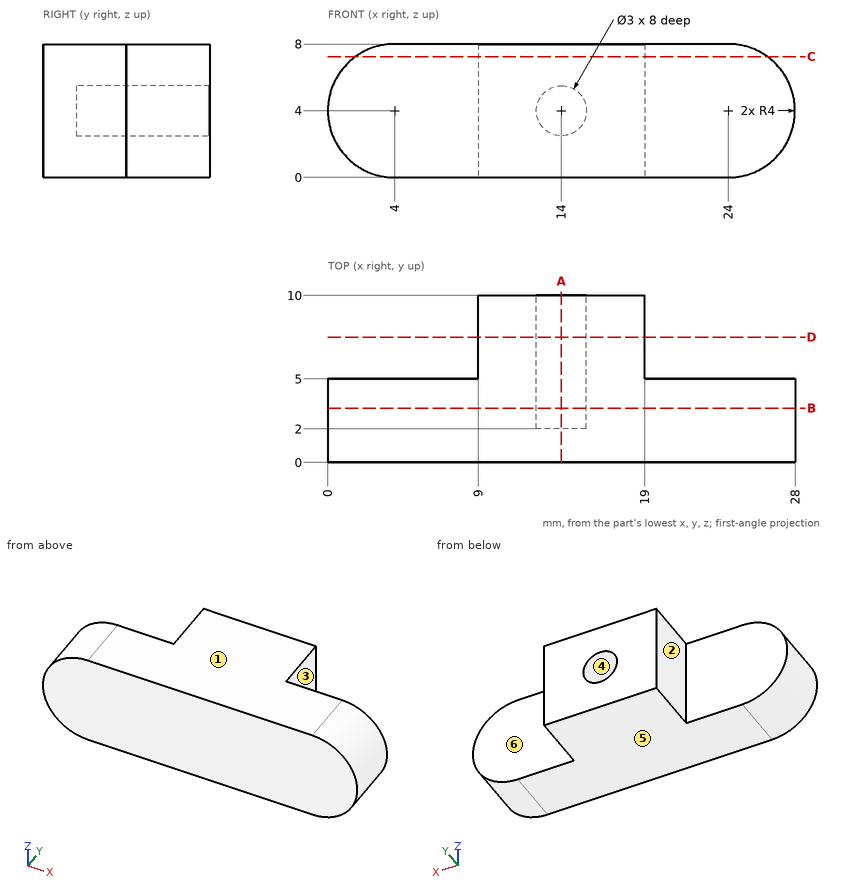
Input: dimensioned drawing with shaded views. Units: mm. Origin: part minimum x, y, z. A direction names the side the tool comes from. Coordinates: 2 decimals unless noted, no trailing zeros. Order: outer loops, then holes, each group sorted by start corner. A loop starts at its lowest first (then second) coordinate and runs counter-clockwise, first axis right, second up. Notation, with made-up numbers: M 58.5,18 L 63.5,18 A26 cw 63.5,48 Z; hole C 4.5,-16 d8. An arc over 180 degrees is marked long. Write each question's results on one line, items separated by ' | '. Start each with the question number.
Item 1: Cut plane D-D (y = 7.5). Return loops of the section in (x, z), and give its area (3 significant figures).
Item 2: Set-up query: the marked faces 1, 2 and 3. Return all of +Z, -Z, +X, -X, +Y, -Y with unobstructed straight access to the full face (end or side cutting, diameter ignored); none if empty.
Item 3: First-contact query: pin 1 Ø3 at (x, z) = (24.5, 2) entering from -Y; pin 2 Ø2.5 at (y, z) = (7, 2.5) entering from -X; pin 3 Ø2.5 at (x, z) = (22, 5) entering from +Y. Flat tips, straight axial feed; report the tip coordinate or a pass-through.
Item 4: Cut plane C-C (z = 7.25). Return loops of the section in (x, y).
Item 5: Line query: probe 1 along X at (y, z) = (7, 4); probe 2 along X at (y, z) = (4, 4); probe 3 along Y at (x, z) = (6.5, 7.5). Output: solid intervals per line, ascending.
Item 6: Cut plane B-B (y = 3.25). Return loops of the section in (x, z), and give its area (3 significant figures).
Item 7: Draft query along Z for the marked faces 4, 5 and 6. Return one class per face: pulls with the +Z half, pulls with the -Z half, needs draft (parallel to the pull), parting line crosses it, or undercut.
Item 8: Cut plane A-A (x = 14). Return loops of the section in (y, z).
Checked values:
1) outline: M 9,0 L 19,0 L 19,8 L 9,8 Z; hole C 14,4 d3 | area: 72.9 mm2
2) face 1: +Z, +X, -X, +Y, -Y | face 2: +Z, -Z, -X, +Y | face 3: +Z, -Z, +X, +Y
3) pin 1: stops at y = 0 | pin 2: stops at x = 9 | pin 3: stops at y = 5
4) outline: M 1.67,0 L 26.33,0 L 26.33,5 L 19,5 L 19,10 L 9,10 L 9,5 L 1.67,5 Z
5) probe 1: x = 9 to 12.5, 15.5 to 19 | probe 2: x = 0 to 12.5, 15.5 to 28 | probe 3: y = 0 to 5
6) outline: M 4,0 L 24,0 A4 ccw 24,8 L 4,8 A4 ccw Z; hole C 14,4 d3 | area: 203 mm2
7) face 4: undercut | face 5: pulls with the -Z half | face 6: needs draft
8) outline: M 0,0 L 10,0 L 10,2.5 L 2,2.5 L 2,5.5 L 10,5.5 L 10,8 L 0,8 Z
